Check sheet for the modelled part. Datum: model origin and axes. Units: mm. A direction names the side the tool comes from. Round coordinates to 2 decimals unless told otherwise and drop trailing zeros. Order: outer loops, then holes, each group sorted by start corner. A loop starts at its lowest first (then second) coordinate and runs counter-clockwise, first axis right, second up.
(1) Depth check by flat-ended pin: pin 1 (1.1 mm diameter, centred on y = 61.5, z = 2.5, fed in from -X); pin 2 (1 mm diameter, centred on x = 62, z = 1.5, fed in from -Y) (3 decimals); pin 3 (1 mm diameter, centred on x = 67, z = 2.5, fed in from +Y). Enter the tip coordinate at first touch or a pass-through.
(2) Sectioned sample at C-C, the plane x = -57. Enter the section's corners in (y, z) (3 decimals).
(3) Mould release check, pull along Y, two halves, no side actions. Record for faces 1 (the flat face through (0, 12, 0)), 2 (the cylindrical face through (2.85, 97.43, 1.57)), 3 (the cylindrical face through (-78.34, -51.77, 1.61)), 4 (the cylindrical face through (88.14, -19.02, 1.57)): released by +Y, released by -Y, zero draft, split by the parting line, or undercut.
(4) Sectioned sample at B-B, the plane x = -17. Enter the section's corners in (y, z) (3 decimals), and give its area (3 significant figures).
(5) Tool access check on faces 5 (the cylindrical face through (28.58, 85.52, 1.57)), 6 (the flat face through (0, 12, 3.175)). Record the directions out of +Z, -Z, +X, -X, +Y, -Y that give a thin tool (end or side, any length) a straight path to the whole face; none if there is none.
(6) Sectioned sample at D-D, the plane z = 0.95. Count the separate pieces of the cut face and the enclosed holes in it, and give its area (3 significant figures).
(7) Thickness scan on probe 1 along X at (y, z) = (-1.5, 2.5); probe 2 along Y at (x, z) = (14, 2) (3 decimals); probe 3 along Y at (x, z) = (41, 2.25) (3 decimals). Record the ranges inside material, lowest first.
(8) Sectioned sample at A-A, the plane y = 2. Enter the section's corners in (x, z) (3 decimals).
```python
from build123d import *

# Parameters (mm, degrees)
SKETCH1_R           = 97.4725
SKETCH1_R_2         = 90.17
BOSS_EXTRUDE1_DEPTH = 3.175
BOSS_EXTRUDE2_START = -3.175
BOSS_EXTRUDE2_DEPTH = 3.175
CIRPATTERN2_COUNT   = 3
CUT_EXTRUDE1_DEPTH  = 138.883491171
BOSS_EXTRUDE5_START = -3.175
SKETCH13_W          = 20.066
SKETCH13_H          = 3.175
BOSS_EXTRUDE5_DEPTH = 3.175
BOSS_EXTRUDE6_START = -3.175
SKETCH17_W          = 20.066
SKETCH17_H          = 3.175
BOSS_EXTRUDE6_DEPTH = 3.175
FILLET1_R           = 6.35
FILLET2_R           = 0.508


with BuildPart() as part:
    # Sketch1 → Boss-Extrude1 (new body)
    with BuildSketch(Plane.XY):
        Circle(SKETCH1_R)
        Circle(SKETCH1_R_2, mode=Mode.SUBTRACT)
    extrude(amount=BOSS_EXTRUDE1_DEPTH)

    # Sketch2 → Boss-Extrude2 (add)
    with BuildSketch(Plane.XY.offset(3.175).offset(BOSS_EXTRUDE2_START)):
        with BuildLine():
            ThreePointArc((-5.291472464, 86.659612676), (0, 83.82), (5.291472464, 86.659612676))
            ThreePointArc((5.291472464, 86.659612676), (7.940261692, 88.923194985), (11.38468318, 89.448409091))
            ThreePointArc((11.38468318, 89.448409091), (0, 90.17), (-11.38468318, 89.448409091))
            ThreePointArc((-11.38468318, 89.448409091), (-7.940261692, 88.923194985), (-5.291472464, 86.659612676))
        make_face()
    boss_extrude2 = extrude(amount=BOSS_EXTRUDE2_DEPTH)

    # Sketch7 → #6 Clearance Hole2 (revolve, cut)
    with BuildSketch(Plane(origin=(0, 90.17, 0), x_dir=(0, 1, 0), z_dir=(1, 0, 0))):
        Polygon((0, 0), (0, 7.490824014), (1.89865, 6.35), (1.89865, 0), align=None)
    f_6_clearance_hole2 = revolve(axis=Axis((0, 90.17, -6.35), (0, 0, 1)), mode=Mode.SUBTRACT)

    # CirPattern2: Boss-Extrude2, #6 Clearance Hole2 ×3 about axis
    cirpattern2_axis = Axis((0, 0, 0), (0, 0, 1))
    add([boss_extrude2.rotate(cirpattern2_axis, i * 360 / CIRPATTERN2_COUNT) for i in range(1, CIRPATTERN2_COUNT)])
    add([f_6_clearance_hole2.rotate(cirpattern2_axis, i * 360 / CIRPATTERN2_COUNT) for i in range(1, CIRPATTERN2_COUNT)], mode=Mode.SUBTRACT)

    # Sketch14 → Cut-Extrude1 (cut, through all)
    with BuildSketch(Plane.XY.offset(3.175)):
        with BuildLine():
            ThreePointArc((-72.403689828, -47.912355915), (-78.441248685, -51.771990171), (-84.687137855, -48.259475113))
            ThreePointArc((-84.687137855, -48.259475113), (6.18e-07, -97.4725), (84.687138467, -48.25947404))
            ThreePointArc((84.687138467, -48.25947404), (78.441249322, -51.771989501), (72.403689828, -47.912355915))
            ThreePointArc((72.403689828, -47.912355915), (73.039614996, -51.33806583), (71.772253011, -54.583629393))
            ThreePointArc((71.772253011, -54.583629393), (0, -90.17), (-71.772253011, -54.583629393))
            ThreePointArc((-71.772253011, -54.583629393), (-73.039614996, -51.33806583), (-72.403689828, -47.912355915))
        make_face()
    extrude(amount=-CUT_EXTRUDE1_DEPTH, mode=Mode.SUBTRACT)

    # Sketch13 → Boss-Extrude5 (add)
    with BuildSketch(Plane.XY.offset(3.175).offset(BOSS_EXTRUDE5_START)):
        with BuildLine():
            Line((-90.0603735, 4.445), (90.0603735, 4.445))
            ThreePointArc((90.0603735, 4.445), (89.697330897, 9.220505951), (89.081243817, 13.97))
            Line((89.081243817, 13.97), (-89.081243817, 13.97))
            ThreePointArc((-89.081243817, 13.97), (-89.697330897, 9.220505951), (-90.0603735, 4.445))
        make_face()
        with Locations((-63.5, 9.2075)):
            Rectangle(SKETCH13_W, SKETCH13_H, mode=Mode.SUBTRACT)
        with Locations((63.5, 9.2075)):
            Rectangle(SKETCH13_W, SKETCH13_H, mode=Mode.SUBTRACT)
    extrude(amount=BOSS_EXTRUDE5_DEPTH)

    # Sketch17 → Boss-Extrude6 (add)
    with BuildSketch(Plane.XY.offset(3.175).offset(BOSS_EXTRUDE6_START)):
        with BuildLine():
            Line((-60.704804382, 66.675), (60.704804382, 66.675))
            ThreePointArc((60.704804382, 66.675), (65.399047227, 62.0773189), (69.746013506, 57.15))
            Line((69.746013506, 57.15), (-69.746013506, 57.15))
            ThreePointArc((-69.746013506, 57.15), (-65.399047227, 62.0773189), (-60.704804382, 66.675))
        make_face()
        with Locations((-41.275, 61.9125)):
            Rectangle(SKETCH17_W, SKETCH17_H, mode=Mode.SUBTRACT)
        with Locations((41.275, 61.9125)):
            Rectangle(SKETCH17_W, SKETCH17_H, mode=Mode.SUBTRACT)
    extrude(amount=BOSS_EXTRUDE6_DEPTH)

    # Fillet1
    fillet1_edges = [part.edges().sort_by_distance(p)[0] for p in [
        (69.746013506, 57.15, 1.5875),
        (60.704804382, 66.675, 1.5875),
        (-60.704804382, 66.675, 1.5875),
        (-69.746013506, 57.15, 1.5875),
        (90.0603735, 4.445, 1.5875),
        (89.081243817, 13.97, 1.5875),
        (-89.081243817, 13.97, 1.5875),
        (-90.0603735, 4.445, 1.5875),
    ]]
    fillet(fillet1_edges, radius=FILLET1_R)

    # Fillet2
    fillet2_edges = [part.edges().sort_by_distance(p)[0] for p in [
        (-51.308, 60.325, 1.5875),
        (-31.242, 60.325, 1.5875),
        (-31.242, 63.5, 1.5875),
        (-51.308, 63.5, 1.5875),
        (31.242, 60.325, 1.5875),
        (51.308, 60.325, 1.5875),
        (51.308, 63.5, 1.5875),
        (31.242, 63.5, 1.5875),
        (-73.533, 7.62, 1.5875),
        (-53.467, 7.62, 1.5875),
        (-53.467, 10.795, 1.5875),
        (-73.533, 10.795, 1.5875),
        (53.467, 7.62, 1.5875),
        (73.533, 7.62, 1.5875),
        (73.533, 10.795, 1.5875),
        (53.467, 10.795, 1.5875),
    ]]
    fillet(fillet2_edges, radius=FILLET2_R)


solid = part.part
```
Derived:
1. pin 1: stops at x = -76.07
1. pin 2: stops at y = 4.445
1. pin 3: stops at y = 71.26
2. outline: (4.445, 0) - (7.62, 0) - (7.62, 3.175) - (4.445, 3.175) - close; (10.795, 0) - (13.97, 0) - (13.97, 3.175) - (10.795, 3.175) - close; (57.15, 0) - (79.069, 0) - (79.069, 3.175) - (57.15, 3.175) - close
3. face 1: zero draft
3. face 2: split by the parting line
3. face 3: released by -Y
3. face 4: undercut
4. outline: (4.445, 0) - (13.97, 0) - (13.97, 3.175) - (4.445, 3.175) - close; (57.15, 0) - (66.675, 0) - (66.675, 3.175) - (57.15, 3.175) - close; (88.553, 0) - (95.979, 0) - (95.979, 3.175) - (88.553, 3.175) - close
4. area: 84.1 mm2
5. face 5: +Z, -Z
5. face 6: +Z, +X, -X, +Y, -Y
6. separate pieces: 1
6. enclosed holes: 9
6. area: 6,020 mm2
7. probe 1: x = -97.46 to -90.14, 90.14 to 97.46
7. probe 2: y = 4.445 to 13.97, 57.15 to 66.675, 89.077 to 96.462
7. probe 3: y = 4.445 to 13.97, 57.15 to 60.325, 63.5 to 66.675, 80.31 to 88.43
8. outline: (-97.452, 0) - (-88.806, 0) - (-88.806, 3.175) - (-97.452, 3.175) - close; (88.806, 0) - (97.452, 0) - (97.452, 3.175) - (88.806, 3.175) - close
